The model under review builds one solid part; all positions refer to its coordinate system, in mm. Round coordinates to 2 decimals unless told otherwise and drop trailing zeros. Write each loop counter-clockwise with the first axis right and the second up, starting at its lowest first coordinate (ties: lowest second). Pieces come first, ordered by that corner, then holes. Notation, with made-up numbers: (66, 29) - (113, 29) arc R23 ccw to (113, 46) - close; hole circle Ø6 at (27.5, 29.25). An arc over 180 degrees is marked (long way). Write each question's results on one line, items separated by ' | '.
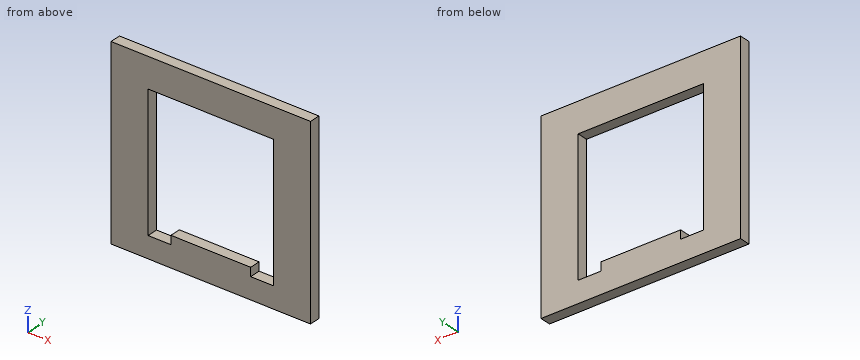
```python
from build123d import *

# Parameters (mm, degrees)
SCHIZZO1_W                   = 70
SCHIZZO1_H                   = 65
ESTRUSIONE_ESTRUSIONE1_DEPTH = 3.76


with BuildPart() as part:
    # Schizzo1 → Estrusione-Estrusione1 (new body)
    with BuildSketch(Plane(origin=(0, 0, 0), x_dir=(1, 0, 0), z_dir=(0, 1, 0))):
        Rectangle(SCHIZZO1_W, SCHIZZO1_H)
        Polygon((-22, -22), (-22, 22), (-22, 25), (-14, 25), (-14, 22), (14, 22), (14, 25), (22, 25), (22, 22), (22, -22), align=None, mode=Mode.SUBTRACT)
    extrude(amount=ESTRUSIONE_ESTRUSIONE1_DEPTH)


solid = part.part
```
Q1. We need section B-B (z = -1). State the section outline as (x, y) points.
Evaluation:
outline: (-35, 0) - (-22, 0) - (-22, 3.76) - (-35, 3.76) - close; (22, 0) - (35, 0) - (35, 3.76) - (22, 3.76) - close
Q2. Insertion check: P1, Ø4, axis at x = 14, z = 21.5, coming from the -Y side. The pin has a flat end and moves straight along its axis. Give the tip position at first contact, or say it passes through.
Evaluation:
P1: stops at y = 0
Q3. We need section C-C (y = 1.75). State the section outline as (x, z) points, plus the area to 3 significant figures.
Evaluation:
outline: (-35, -32.5) - (35, -32.5) - (35, 32.5) - (-35, 32.5) - close; hole (-22, -25) - (-14, -25) - (-14, -22) - (14, -22) - (14, -25) - (22, -25) - (22, 22) - (-22, 22) - close | area: 2,570 mm^2
Q4. We need section A-A (x = -20). State the section outline as (y, z) points, plus the area to 3 significant figures.
Evaluation:
outline: (0, -32.5) - (3.76, -32.5) - (3.76, -25) - (0, -25) - close; (0, 22) - (3.76, 22) - (3.76, 32.5) - (0, 32.5) - close | area: 67.7 mm^2
Q5. For probe 1 along Z at (x, y) = (11, 2.7); probe 2 along X at (y, z) = (0.4, -11), list the stretches that pass through material, from the lowest coordinate up.
Evaluation:
probe 1: z = -32.5 to -22, 22 to 32.5 | probe 2: x = -35 to -22, 22 to 35
